Check sheet for the modelled part. Datum: model origin and axes. Units: mm. A direction names the side the tool comes from. Coordinates: 2 decimals unless noted, no trailing zeros. Write each loop counter-clockwise with the first axis right and the second up, starting at its lowest first coordinate (ties: lowest second). Pieces come first, ordered by that corner, then holes. Notation, with made-up numbers: (43, 24) - (69, 24) arc R18 ccw to (69, 29) - close; hole circle Ø7 at (64, 27.5). An arc over 180 degrees is marked (long way). Write each question's results on one line, items separated by ' | '.
from build123d import *

# Parameters (mm, degrees)
SKETCH_1_W          = 80
SKETCH_1_H          = 55
EXTRUDE_1_DEPTH     = 20
SKETCH_2_W          = 15
SKETCH_2_H          = 10
EXTRUDE_2_DEPTH     = 10
SKETCH_3_W          = 8.5
SKETCH_3_H          = 15
EXTRUDE_3_DEPTH     = 5
SKETCH_4_W          = 60
SKETCH_4_H          = 10
EXTRUDE_4_DEPTH     = 10
SKETCH_5_W          = 60
SKETCH_5_H          = 8.5
EXTRUDE_5_DEPTH     = 5
SKETCH_6_W          = 96
SKETCH_6_H          = 20
EXTRUDE_6_DEPTH     = 2.5
SKETCH_7_W          = 96
SKETCH_7_H          = 55
EXTRUDE_8_DEPTH     = 2.5
FILLET_1_R          = 2
CUT_EXTRUDE_1_DEPTH = 2.5


with BuildPart() as part:
    # 草图1 → 凸台-拉伸1 (new body)
    with BuildSketch(Plane(origin=(0, 0, 0), x_dir=(1, 0, 0), z_dir=(0, 1, 0))):
        Rectangle(SKETCH_1_W, SKETCH_1_H)
    extrude(amount=EXTRUDE_1_DEPTH)

    # 草图2 → 凸台-拉伸2 (add)
    with BuildSketch(Plane(origin=(40, 0, 0), x_dir=(0, 0, -1), z_dir=(1, 0, 0))):
        with Locations((-5, 13)):
            Rectangle(SKETCH_2_W, SKETCH_2_H)
    extrude(amount=EXTRUDE_2_DEPTH)

    # 草图3 → 凸台-拉伸3 (add)
    with BuildSketch(Plane(origin=(0, 18, 0), x_dir=(1, 0, 0), z_dir=(0, 1, 0))):
        with Locations((45.75, -5)):
            Rectangle(SKETCH_3_W, SKETCH_3_H)
    extrude(amount=EXTRUDE_3_DEPTH)

    # 草图4 → 凸台-拉伸4 (add)
    with BuildSketch(Plane.XY.offset(27.5)):
        with Locations((0, 13)):
            Rectangle(SKETCH_4_W, SKETCH_4_H)
    extrude(amount=EXTRUDE_4_DEPTH)

    # 草图5 → 凸台-拉伸5 (add)
    with BuildSketch(Plane(origin=(0, 18, 0), x_dir=(1, 0, 0), z_dir=(0, 1, 0))):
        with Locations((0, -33.25)):
            Rectangle(SKETCH_5_W, SKETCH_5_H)
    extrude(amount=EXTRUDE_5_DEPTH)

    # 草图6 → 凸台-拉伸6 (add)
    with BuildSketch(Plane(origin=(0, 0, -27.5), x_dir=(-1, 0, 0), z_dir=(0, 0, -1))):
        with Locations((0, 10)):
            Rectangle(SKETCH_6_W, SKETCH_6_H)
    extrude(amount=-EXTRUDE_6_DEPTH)

    # 草图7 → 凸台-拉伸8 (add)
    with BuildSketch(Plane.XZ):
        Rectangle(SKETCH_7_W, SKETCH_7_H)
    extrude(amount=EXTRUDE_8_DEPTH)

    # 圆角1
    fillet_1_edges = [part.edges().sort_by_distance(p)[0] for p in [
        (48, 20, -26.25),
        (44, 0, -25),
        (-44, 0, -25),
        (-48, 20, -26.25),
        (-48, -1.25, 27.5),
        (48, -1.25, 27.5),
        (0, -2.5, -27.5),
    ]]
    fillet(fillet_1_edges, radius=FILLET_1_R)

    # 草图8 → 切除-拉伸1 (cut)
    with BuildSketch(Plane.XZ.offset(2.5)):
        with BuildLine():
            Line((-48, -3), (-43.25, -3))
            ThreePointArc((-43.25, -3), (-41, -0.75), (-43.25, 1.5))
            Line((-43.25, 1.5), (-48, 1.5))
            Line((-48, 1.5), (-48, -3))
        make_face()
        with BuildLine():
            Line((48, 1.5), (48, -3))
            Line((48, -3), (43.25, -3))
            ThreePointArc((43.25, -3), (41, -0.75), (43.25, 1.5))
            Line((43.25, 1.5), (48, 1.5))
        make_face()
    extrude(amount=-CUT_EXTRUDE_1_DEPTH, mode=Mode.SUBTRACT)


solid = part.part
1. Sectioned sample at B-B (z = -5.5). Record the cut outline in (x, y).
Values follow:
outline: (-48, -2.5) - (48, -2.5) - (48, 0) - (40, 0) - (40, 20) - (-40, 20) - (-40, 0) - (-48, 0) - close
2. Sectioned sample at A-A (x = -0.5). Record the cut outline in (y, z).
Values follow:
outline: (-2.5, -25.5) arc R2 ccw to (-0.5, -27.5) - (20, -27.5) - (20, 27.5) - (18, 27.5) - (18, 29) - (23, 29) - (23, 37.5) - (8, 37.5) - (8, 27.5) - (-2.5, 27.5) - close
3. Material ranges on L1, parallel to Z at x = 15.5, y = 0.5; L2, parallel to Y at x = -11, z = -20; L3, parallel to Y at x = 42, z = -21.5, recorded low to high. Write a range as [from, to].
Values follow:
L1: z = [-27.5, 27.5] | L2: y = [-2.5, 20] | L3: y = [-2.5, 0]
4. Go/stop test with flat-tipped pins: pin 1 (0.8 mm diameter, centred on x = 0.5, z = 28.5, fed in from +Y); pin 2 (1.2 mm diameter, centred on x = 46.5, y = -1.5, fed in from +Z); pin 3 (4 mm diameter, centred on y = 21, z = 4.5, fed in from -X). Record where each tip stops, or that it passes through.
Values follow:
pin 1: stops at y = 18 | pin 2: stops at z = 27.5 | pin 3: stops at x = -40
5. Draft check along X on faces 4 (the flat face through (44, 0, 3)), 5 (the flat face through (41.5, 20, 5)), 6 (the cylindrical face through (-41, -1.3, -0.8)), 7 (the cylindrical face through (47.43, -1.27, 26.9)). Enter one of: pulls with the +X half, pulls with the -X half, needs draft (parallel to the pull), parting line crosses it, or undercut.
Values follow:
face 4: needs draft | face 5: undercut | face 6: pulls with the -X half | face 7: pulls with the +X half
6. Access from +Z, -Z, +X, -X, +Y, -Y to the whole of each face (thin tool, end or side, straight path). Record for faces 1 (the flat face through (48, -1, -21)), 2 (the flat face through (45, 15, -2.5)), 3 (the flat face through (-44, 0, 3)).
Values follow:
face 1: -Z, +X, +Y, -Y | face 2: +X, +Y | face 3: +Z, -X, +Y
7. Sectioned sample at D-D (x = -31). Record the cut outline in (y, z), then the cut area to 3 significant figures.
Values follow:
outline: (-2.5, -25.5) arc R2 ccw to (-0.5, -27.5) - (20, -27.5) - (20, 27.5) - (-2.5, 27.5) - close | area: 1,240 mm^2
8. Sectioned sample at C-C (y = 9.5). Record the cut outline in (x, z).
Values follow:
outline: (-48, -27.5) - (48, -27.5) - (48, -25) - (40, -25) - (40, -2.5) - (50, -2.5) - (50, 12.5) - (40, 12.5) - (40, 27.5) - (30, 27.5) - (30, 37.5) - (-30, 37.5) - (-30, 27.5) - (-40, 27.5) - (-40, -25) - (-48, -25) - close
